Part print with two shaded views. Sizes in mm from the minimum x, y, z corner. Round coordinates to 2 decimals unless told otherwise and drop trailing zeros. Order: outer loops, then holes, each group sorted by start corner. A loop starts at its lowest first (then second) coordinate and runs counter-clockwise, first axis right, second up. Notation, with made-up numbers: (-3, -32.75) -> (25, -32.75) arc R27 ccw to (25, -16.75) -> close; hole circle Ø2 at (86.5, -13.5). An arc over 180 degrees is marked (long way). Answer as a JSON object with one key per item and string values.
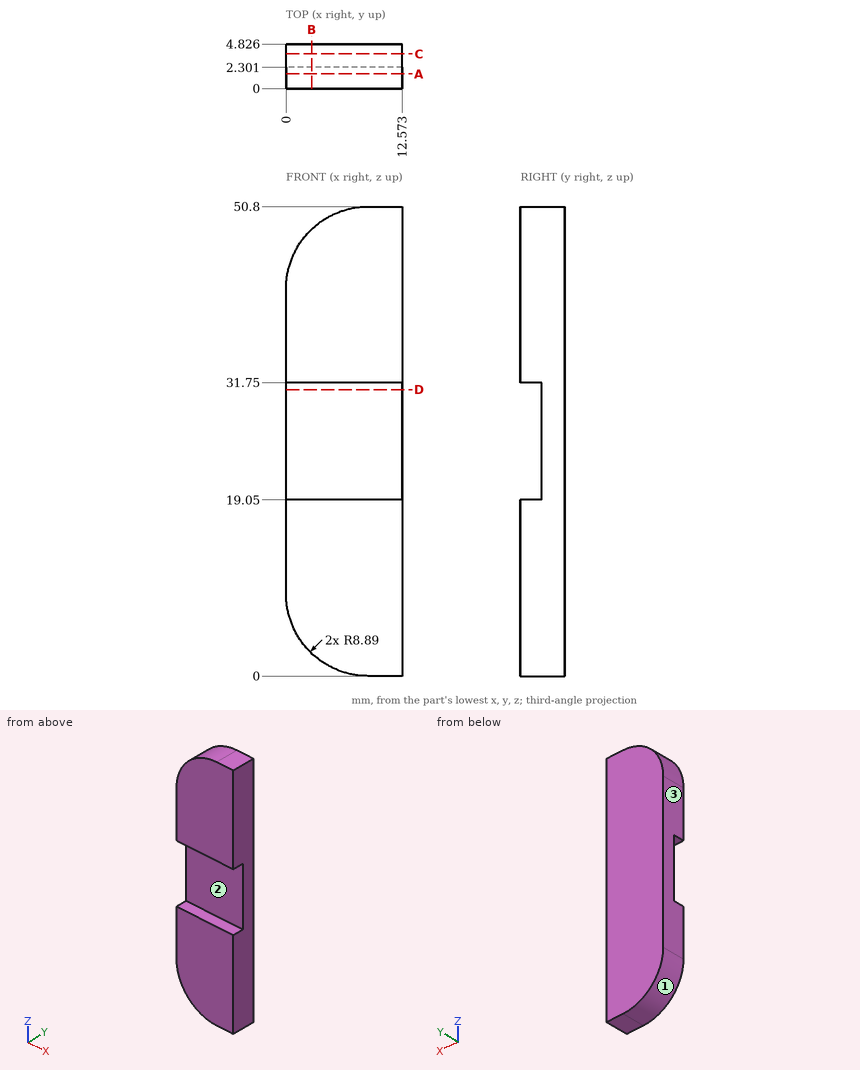
1) Cut at A-A, the plane y = 1.6. Give the cut face in (x, z), plus the area to 3 significant figures.
Checked values:
{"outline": "(0, 8.89) arc R8.89 ccw to (8.89, 0) -> (12.57, 0) -> (12.57, 19.05) -> (0, 19.05) -> close; (0, 31.75) -> (12.57, 31.75) -> (12.57, 50.8) -> (8.89, 50.8) arc R8.89 ccw to (0, 41.91) -> close", "area": "445 mm²"}
2) Flat gauge pins, fed straight in: pin 1 Ø1 at (x, y) = (6, 4) entering from -Z; pin 2 Ø1 at (x, y) = (1.5, 3) entering from +Z; pin 3 Ø1 at (x, y) = (4.5, 3) entering from -Z. Where does each tip first touch, or does it go through?
Checked values:
{"pin 1": "stops at z = 0.33", "pin 2": "stops at z = 47.53", "pin 3": "stops at z = 0.9"}
3) Cut at C-C, the plane y = 3.75. Give the cut face in (x, z).
Checked values:
{"outline": "(0, 8.89) arc R8.89 ccw to (8.89, 0) -> (12.57, 0) -> (12.57, 50.8) -> (8.89, 50.8) arc R8.89 ccw to (0, 41.91) -> close"}
4) Cut at B-B, the plane x = 2.75. Give the cut face in (y, z), plus the area to 3 significant figures.
Checked values:
{"outline": "(0, 2.46) -> (4.83, 2.46) -> (4.83, 48.34) -> (0, 48.34) -> (0, 31.75) -> (2.3, 31.75) -> (2.3, 19.05) -> (0, 19.05) -> close", "area": "192 mm²"}
5) Pull direction Z, two halves, no side cores. Call the marked faces 1, 2 and 3: pulls with the +Z half, pulls with the -Z half, needs draft (parallel to the pull), parting line crosses it, or undercut.
Checked values:
{"face 1": "pulls with the -Z half", "face 2": "undercut", "face 3": "needs draft"}
6) Probe L1, parallel to Y at x = 8.75, z = 29; L2, parallel to Z at x = 6, y = 2.1; L3, parallel to Z at x = 7, y = 0.45. List the from-to ranges inside material, lowest first. Write a range as from..to.
Checked values:
{"L1": "y = 2.3..4.83", "L2": "z = 0.48..19.05, 31.75..50.32", "L3": "z = 0.2..19.05, 31.75..50.6"}
7) Cut at D-D, the plane z = 31. Give the cut face in (x, y).
Checked values:
{"outline": "(0, 2.3) -> (12.57, 2.3) -> (12.57, 4.83) -> (0, 4.83) -> close"}
